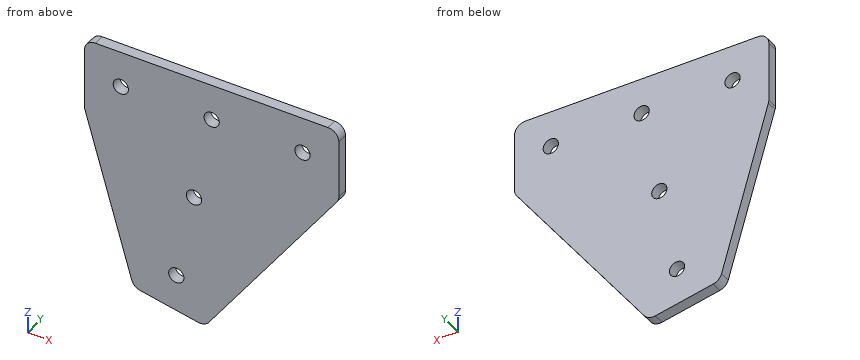
from build123d import *

# Parameters (mm, degrees)
SKETCH_1_W      = 70
SKETCH_1_H      = 20
SKETCH_1_R      = 2.1
EXTRUDE_1_DEPTH = 3
FILLET_1_R      = 3


with BuildPart() as part:
    # 草图1 → 凸台-拉伸1 (new body)
    # profile 1 of 4: a face of its own
    with BuildSketch(Plane(origin=(0, 0, 0), x_dir=(1, 0, 0), z_dir=(0, 1, 0))):
        Polygon((-1.865732489, 60.799005274), (8.211170098, 10), (35, 10), align=None)
    # profile 2 of 4: a face of its own
    with BuildSketch(Plane(origin=(0, 0, 0), x_dir=(1, 0, 0), z_dir=(0, 1, 0))):
        Rectangle(SKETCH_1_W, SKETCH_1_H)
        with Locations(Location((-25, 0, 0), (0, 0, 270))):
            Circle(SKETCH_1_R, mode=Mode.SUBTRACT)
        with Locations(Location((25, 0, 0), (0, 0, 270))):
            Circle(SKETCH_1_R, mode=Mode.SUBTRACT)
        with Locations(Location((0, 0, 0), (0, 0, 270))):
            Circle(SKETCH_1_R, mode=Mode.SUBTRACT)
    # profile 3 of 4: a face of its own
    with BuildSketch(Plane(origin=(0, 0, 0), x_dir=(1, 0, 0), z_dir=(0, 1, 0))):
        Polygon((-35, 10), (-12.178532268, 10), (-21.48347839, 56.907470127), align=None)
    # profile 4 of 4: a face of its own
    with BuildSketch(Plane(origin=(0, 0, 0), x_dir=(1, 0, 0), z_dir=(0, 1, 0))):
        Polygon((-12.178532268, 10), (8.211170098, 10), (-1.865732489, 60.799005274), (-21.48347839, 56.907470127), align=None)
        with Locations(Location((-4.864418933, 24.522182375, 0), (0, 0, 270))):
            Circle(SKETCH_1_R, mode=Mode.SUBTRACT)
        with Locations(Location((-9.728837866, 49.04436475, 0), (0, 0, 270))):
            Circle(SKETCH_1_R, mode=Mode.SUBTRACT)
    extrude(amount=EXTRUDE_1_DEPTH)

    # 圆角1
    fillet_1_edges = [part.edges().sort_by_distance(p)[0] for p in [
        (-1.865732489, 1.5, -60.799005274),
        (35, 1.5, -10),
        (35, 1.5, 10),
        (-35, 1.5, 10),
        (-35, 1.5, -10),
        (-21.48347839, 1.5, -56.907470127),
    ]]
    fillet(fillet_1_edges, radius=FILLET_1_R)


solid = part.part
Part model, mm, in its own coordinate system. Give positions to 0.01 mm unless a question says otherwise; leave off trailing zeros. Loops run counter-clockwise (first coordinate to the right, second up) from the corner with the lowest first, then second, coordinate; pieces in that order, holes last. Notation, with made-up numbers: (82, 63) -> (96, 63) arc R11 ccw to (96, 77) -> close; hole circle Ø9 at (28.5, -17.75). An arc over 180 degrees is marked (long way). Write each question's results on one line, items separated by ' | '. Start each with the question number.
Q1. Band-saw the part on B-B on x = 25. List the corners of the cut face in (y, z).
Q2. Wall check: L1, parallel to X at y = 1.25, z = 0; L2, parallel to Z at x = 25.5, y = 2.65; L3, parallel to Z at x = -5, y = 2.1. Give the ranges that are in metal, low to high.
Q3. Band-saw the part on C-C on y = 2.5. List the corners of the cut face in (x, z).
Q4. Band-saw the part on D-D on x = -25. List the corners of the cut face in (y, z), plus the area to 3 significant figures.
Q5. Band-saw the part on A-A on z = 0. List the corners of the cut face in (x, y).
Results are:
1) outline: (0, -23.78) -> (3, -23.78) -> (3, -2.1) -> (0, -2.1) -> close; (0, 2.1) -> (3, 2.1) -> (3, 10) -> (0, 10) -> close
2) L1: x = -35 to -27.1, -22.9 to -2.1, 2.1 to 22.9, 27.1 to 35 | L2: z = -23.09 to -2.04, 2.04 to 10 | L3: z = -60.18 to -26.62, -22.43 to 10
3) outline: (-35, -9.58) arc R3 ccw to (-34.88, -10.41) -> (-21.99, -55.15) arc R3 ccw to (-19.69, -57.26) -> (-3.75, -60.43) arc R3 ccw to (-0.74, -59.24) -> (34.43, -10.79) arc R3 ccw to (35, -9.03) -> (35, 7) arc R3 ccw to (32, 10) -> (-32, 10) arc R3 ccw to (-35, 7) -> close; hole circle Ø4.2 at (-25, 0); hole circle Ø4.2 at (-9.73, -49.04); hole circle Ø4.2 at (-4.86, -24.52); hole circle Ø4.2 at (0, 0); hole circle Ø4.2 at (25, 0)
4) outline: (0, -44.7) -> (3, -44.7) -> (3, -2.1) -> (0, -2.1) -> close; (0, 2.1) -> (3, 2.1) -> (3, 10) -> (0, 10) -> close | area: 152 mm²
5) outline: (-35, 0) -> (-27.1, 0) -> (-27.1, 3) -> (-35, 3) -> close; (-22.9, 0) -> (-2.1, 0) -> (-2.1, 3) -> (-22.9, 3) -> close; (2.1, 0) -> (22.9, 0) -> (22.9, 3) -> (2.1, 3) -> close; (27.1, 0) -> (35, 0) -> (35, 3) -> (27.1, 3) -> close
